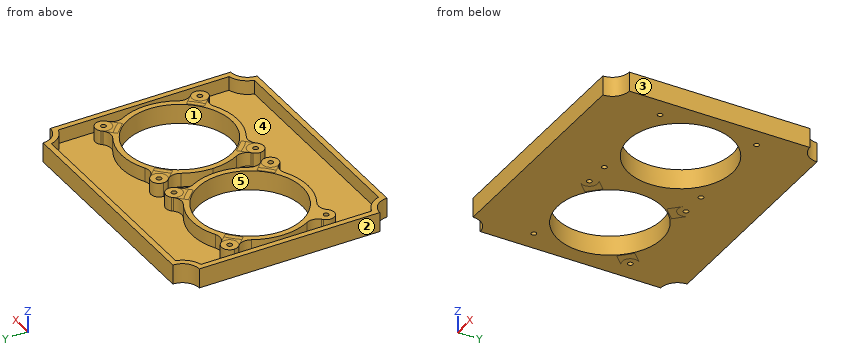
Autodesk Fusion 360 part; units mm, degrees
sketch "Sketch1" plane through (0, 0, 0) normal (0, 0, 1) x (1, 0, 0)
  line L0 (69.35, 57.35) -> (-69.35, 57.35)
  line L1 (-69.35, 57.35) -> (-69.35, -57.35)
  line L2 (-69.35, -57.35) -> (69.35, -57.35)
  line L3 (69.35, -57.35) -> (69.35, 57.35)
  line L4 (69.35, 57.35) -> (-69.35, -57.35) construction
  line L5 (-69.35, 57.35) -> (69.35, -57.35) construction
  circle A0 centre (-69.35, -57.35) radius 9
  circle A1 centre (-69.35, 57.35) radius 9
  circle A2 centre (69.35, 57.35) radius 9
  circle A3 centre (69.35, -57.35) radius 9
  line L6 (-69.35, 0) -> (69.35, 0) construction
  line L7 (0, 57.35) -> (0, -57.35) construction
  dimension "d1" = 138.7
  dimension "d2" = 114.7
  dimension "d3" = 18
  dimension "d4" = 18
  dimension "d5" = 18
  dimension "d6" = 18
extrude "Extrude1" add sketch "Sketch1" along normal blind 10.5 contours L0 L1 L2 L3 A0 A1 A2 A3
sketch "Sketch2" plane through (0, 0, 10.5) normal (0, 0, 1) x (-1, 0, 0)
  line L0 (69.35, -48.35) -> (69.35, 48.35)
  arc A0 (60.35, 57.35) -> (69.35, 48.35) centre (69.35, 57.35) ccw
  line L1 (60.35, 57.35) -> (-60.35, 57.35)
  arc A1 (-69.35, 48.35) -> (-60.35, 57.35) centre (-69.35, 57.35) ccw
  line L2 (-69.35, 48.35) -> (-69.35, -48.35)
  arc A2 (-60.35, -57.35) -> (-69.35, -48.35) centre (-69.35, -57.35) ccw
  line L3 (-60.35, -57.35) -> (60.35, -57.35)
  arc A3 (69.35, -48.35) -> (60.35, -57.35) centre (69.35, -57.35) ccw
  line L4 (69.35, 0) -> (-69.8, 0) construction
  line L5 (0, -57.35) -> (0, 57.35) construction
  circle A4 centre (32.6, 0) radius 28
  circle A5 centre (-33, 0) radius 28
  line L6 (-5, -37.1014) -> (-5, 36.8081) construction
  line L7 (4.6, -36.5148) -> (4.6, 40.6209) construction
  line L8 (-61, -35.195) -> (-61, 33.5819) construction
  line L9 (60.6, -36.0749) -> (60.6, 31.9688) construction
  line L10 (53.819, 28) -> (8.2122, 28) construction
  line L11 (-10.8518, 28) -> (-54.5522, 28) construction
  line L12 (6.75, -25.85) -> (58.45, -25.85) construction
  line L13 (58.45, -25.85) -> (58.45, 25.85) construction
  line L14 (58.45, 25.85) -> (6.75, 25.85) construction
  line L15 (6.75, 25.85) -> (6.75, -25.85) construction
  line L16 (6.75, -25.85) -> (58.45, 25.85) construction
  line L17 (58.45, -25.85) -> (6.75, 25.85) construction
  line L18 (-58.85, -25.85) -> (-7.15, -25.85) construction
  line L19 (-7.15, -25.85) -> (-7.15, 25.85) construction
  line L20 (-7.15, 25.85) -> (-58.85, 25.85) construction
  line L21 (-58.85, 25.85) -> (-58.85, -25.85) construction
  line L22 (-58.85, -25.85) -> (-7.15, 25.85) construction
  line L23 (-7.15, -25.85) -> (-58.85, 25.85) construction
  circle A6 centre (58.45, -25.85) radius 1.35
  circle A7 centre (6.75, 25.85) radius 1.35
  circle A8 centre (6.75, -25.85) radius 1.35
  circle A9 centre (-7.15, -25.85) radius 1.35
  circle A10 centre (-7.15, 25.85) radius 1.35
  circle A11 centre (-58.85, 25.85) radius 1.35
  circle A12 centre (-58.85, -25.85) radius 1.35
  circle A13 centre (58.45, 25.85) radius 1.35
  line L24 (-69.35, 30) -> (70.3, 30)
  line L25 (69.35, -30) -> (-69.35, -30)
  line L26 (51.0272, -28) -> (12.0546, -28) construction
  point P0 (32.6, 0)
  point P1 (-33, 0)
  dimension "d9" = 56
  dimension "d10" = 56
  dimension "d11" = 65.6
  dimension "d12" = 9.6
  dimension "d16" = 29.35
  dimension "d17" = 51.7
  dimension "d18" = 51.7
  dimension "d19" = 51.7
  dimension "d20" = 51.7
  dimension "d21" = 2.7
  dimension "d22" = 2.7
  dimension "d23" = 2.7
  dimension "d24" = 2.7
  dimension "d25" = 2.7
  dimension "d26" = 2.7
  dimension "d27" = 2.7
  dimension "d28" = 2.7
  dimension "d31" = 2
  dimension "d32" = 2
extrude "Extrude2" cut sketch "Sketch2" against normal up to surface (10.5 mm away) contours A4 | A5 | A6 | A7 | A8 | A9 | A10 | A11 | A12 | A13
shell "Shell1" thickness 3 removed faces 1 at (-2.25, -47.3, 10.5)
sketch "Sketch3" plane through (0, 0, 10.5) normal (0, 0, 1) x (-1, 0, 0)
  circle A0 centre (58.45, 25.85) radius 4.35
  circle A1 centre (58.45, 25.85) radius 1.35
  line L0 (96.2828, -12.0828) -> (58.4, 25.8)
  line L1 (58.4, 25.8) -> (37.8385, 46.3615)
  line L2 (76.0799, 25.8) -> (20.4357, 25.8) construction
  line L3 (55.3241, 28.8759) -> (49.6672, 23.2191)
  line L4 (61.4759, 22.7241) -> (55.8191, 17.0672)
  line L5 (55.8191, 17.0672) -> (49.6672, 23.2191)
  dimension "d34" = 45
  dimension "d35" = 8
  dimension "d36" = 8
extrude "Extrude3" add sketch "Sketch3" against normal up to surface (10.5 mm away) contours A0 L3 L4 L5
fillet "Fillet1" radius 6 2 edges at (-51.2275, -24.7793, 6.75) (-57.3793, -18.6275, 6.75)
pattern_circular "C-Pattern1" count 4 over 360 about axis through (-32.6, 0, -2.1) along (0, 0, 1) of "Extrude3", "Fillet1"
sketch "Sketch4" plane through (0, 0, 10.5) normal (0, 0, 1) x (-1, 0, 0)
  circle A0 centre (-7.15, 25.85) radius 4.35
  circle A1 centre (-7.15, 25.85) radius 1.35
  line L0 (-27.2826, 33.6671) -> (20.0548, 33.6671) construction
  line L1 (-7.15, 25.85) -> (-21.4201, 40.1201) construction
  line L2 (-7.15, 25.85) -> (1.607, 17.093) construction
  line L3 (-10.2259, 28.9259) -> (-15.8828, 23.2691)
  line L4 (-4.0741, 22.7741) -> (-9.7309, 17.1172)
  line L5 (-9.7309, 17.1172) -> (-15.8828, 23.2691)
  dimension "d43" = 45
  dimension "d44" = 8
  dimension "d45" = 8
extrude "Extrude4" add sketch "Sketch4" against normal up to surface (7.5 mm away) contours A0 L3 L4 L5
fillet "Fillet2" radius 6 2 edges at (14.3725, -24.7793, 6.75) (8.2207, -18.6275, 6.75)
pattern_circular "C-Pattern2" count 4 over 360 about axis through (33, 0, -2.1) along (0, 0, 1) of "Extrude4", "Fillet2"
The listing builds one solid part. Answer for the finished solid, in the listing's coordinates (mm). Face numbers are marked on the shaded views. A direction names the side the tool comes from. Give positions to 0.01 mm unless a question says otherwise; leave off trailing zeros. Order: outer loops, then holes, each group sorted by start corner. A loop starts at its lowest first (then second) coordinate and runs counter-clockwise, first axis right, second up. Notation, with made-up numbers: (-39.5, 30) -> (-21.5, 30) arc R17 ccw to (-21.5, 62) -> close; hole circle Ø2 at (14, 84). An arc over 180 degrees is marked (long way). One line per item, written item: value.
1) Find section C-C, the plane z = 6.75. Count the separate pieces of the cut face and the enclosed holes in it, plus the area to 3 significant figures.
Reported:
separate pieces: 3
enclosed holes: 11
area: 3,200 mm^2
2) Find the intervals of material crossed by line 1 (Y direction, x = -28, z = 5.25); line 2 (X direction, y = 1.5, z = 7.75); line 3 (Y direction, x = -17, z = 5.75), in increasing order.
Reported:
line 1: y = -57.35 to -54.35, -30.66 to -27.62, 27.62 to 30.66, 54.35 to 57.35
line 2: x = -69.35 to -66.35, -63.56 to -60.56, -4.64 to -1.64, 2.04 to 5.04, 60.96 to 63.96, 66.35 to 69.35
line 3: y = -57.35 to -54.35, -26.85 to -23.25, 23.25 to 26.85, 54.35 to 57.35
3) Find section A-A, the plane x = -32.6. Determine the outline of the cut face in (y, z).
Reported:
outline: (-57.35, 0) -> (-28, 0) -> (-28, 10.5) -> (-31, 10.5) -> (-31, 3) -> (-54.35, 3) -> (-54.35, 10.5) -> (-57.35, 10.5) -> close; (28, 0) -> (57.35, 0) -> (57.35, 10.5) -> (54.35, 10.5) -> (54.35, 3) -> (31, 3) -> (31, 10.5) -> (28, 10.5) -> close
4) Find section D-D, the plane y = -42. Determine the outline of the cut face in (x, z).
Reported:
outline: (-69.35, 0) -> (69.35, 0) -> (69.35, 10.5) -> (66.35, 10.5) -> (66.35, 3) -> (-66.35, 3) -> (-66.35, 10.5) -> (-69.35, 10.5) -> close
5) Determine the mould class of the marked faces 1, 2 and 3 for opening direction X: pulls with the +X half, pulls with the -X half, needs draft (parallel to the pull), parting line crosses it, or undercut.
Reported:
face 1: undercut
face 2: pulls with the -X half
face 3: pulls with the +X half
6) Find section B-B, the plane y = 9. Determine the outline of the cut face in (x, z).
Reported:
outline: (-69.35, 0) -> (-59.11, 0) -> (-59.11, 10.5) -> (-62.26, 10.5) -> (-62.26, 3) -> (-66.35, 3) -> (-66.35, 10.5) -> (-69.35, 10.5) -> close; (-6.09, 0) -> (6.49, 0) -> (6.49, 10.5) -> (3.34, 10.5) -> (3.34, 3) -> (-2.94, 3) -> (-2.94, 10.5) -> (-6.09, 10.5) -> close; (59.51, 0) -> (69.35, 0) -> (69.35, 10.5) -> (66.35, 10.5) -> (66.35, 3) -> (62.66, 3) -> (62.66, 10.5) -> (59.51, 10.5) -> close
7) A tool of negligible diameter and unlimited length cuts with its end or side. For the marked faces 4 and 5, from which of +Z, -Z, +X, -X, +Y, -Y can it reach the whole face along a straight path? Write none if from no direction.
Reported:
face 4: +Z
face 5: +Z, -Z
